Source: CAD feature listing. Evaluate the final solid. Frame: model axes, mm. Face numbers are marked on the shaded views. Coordinates: 2 decimals unless noted, no trailing zeros. Order: outer loops, then holes, each group sorted by start corner. A loop starts at its lowest first (then second) coordinate and runs counter-clockwise, first axis right, second up. Notation, with made-up numbers: (-12, 83) -> (1, 83) arc R11 ccw to (1, 87) -> close; hole circle Ø1 at (-15, -26). An arc over 180 degrees is marked (long way). Write item = value, one per line. Start each with the question number.
Item 1: Section query A-A (x = 0). Output: boundary loops of the cut face in (y, z).
Item 2: Contact query for flat-ended pins moving along their axis: pin 1 (5 mm diameter, centred on x = -3, y = 6.5, fed in from +Z); pin 2 (1.5 mm diameter, centred on x = 11, z = -13.5, fed in from -Y); pin 3 (3 mm diameter, centred on y = -3, z = -15.5, fed in from -X); pin 4 (6 mm diameter, centred on x = -13.5, z = -35, fed in from -Y). Output: stop coordinate, or through.
Item 3: Section query D-D (y = 0). Output: boundary loops of the cut face in (x, z).
Item 4: Mould query, pull axis X, two halves, no side actions, for the marked faces 1, 2 and 3. Classes: released by +X, released by -X, zero draft, split by the parting line, or undercut.
Item 5: Section query B-B (x = 24). Output: boundary loops of the cut face in (y, z), then the cut area to 3 significant figures.
Item 6: Ray query, line 1 along Y through (x, z) = (0, -54); line 2 along X through (y, z) = (12, -39); line 3 along X through (y, z) = (-4.5, -46). Return the intervals inside material, ascending. Write a range as [from, to].
Item 7: Section query C-C (z = -10). Output: boundary loops of the cut face in (x, y).
```python
from build123d import *

# Parameters (mm, degrees)
SKETCH4_W          = 60
SKETCH4_H          = 30
CUT_EXTRUDE1_REACH = 75.485
SKETCH6_W          = 42
SKETCH6_H          = 5
CIRPATTERN3_COUNT  = 6


with BuildPart() as part:
    # Sketch4 → Revolve1 (revolve)
    with BuildSketch(Plane(origin=(0, 0, 0), x_dir=(0, 0, -1), z_dir=(1, 0, 0)), mode=Mode.PRIVATE) as revolve1_sk:
        with Locations((30, 15)):
            Rectangle(SKETCH4_W, SKETCH4_H)
    revolve(revolve1_sk.sketch.rotate(Axis((0, 0, 24.398391619), (0, 0, -1)), 90), axis=Axis((0, 0, 24.398391619), (0, 0, -1)))

    # Sketch5 → Cut-Revolve1 (revolve, cut)
    with BuildSketch(Plane(origin=(0, 0, 0), x_dir=(0, 0, -1), z_dir=(1, 0, 0)), mode=Mode.PRIVATE) as cut_revolve1_sk:
        Polygon((0, 0), (0, 19.816349035), (50, 11), (60, 11), (60, 0), align=None)
    revolve(cut_revolve1_sk.sketch.rotate(Axis((0, 0, 8.48865663), (0, 0, -1)), 90), axis=Axis((0, 0, 8.48865663), (0, 0, -1)), mode=Mode.SUBTRACT)

    # Sketch6 → Cut-Extrude1 (cut, up to next)
    with BuildSketch(Plane(origin=(0, 0, 0), x_dir=(0, 0, -1), z_dir=(1, 0, 0)), mode=Mode.PRIVATE) as cut_extrude1_sk1:
        with Locations((21, 0)):
            Rectangle(SKETCH6_W, SKETCH6_H)
    cut_extrude1_tool1 = extrude(cut_extrude1_sk1.sketch, amount=CUT_EXTRUDE1_REACH, mode=Mode.PRIVATE) & part.part
    cut_extrude1 = cut_extrude1_tool1.solids().sort_by_distance((0, 0, -21))[0]
    add(cut_extrude1, mode=Mode.SUBTRACT)

    # CirPattern3: Cut-Extrude1 ×6 about axis
    cirpattern3_axis = Axis((0, 0, 0), (0, 0, 1))
    for i in range(1, CIRPATTERN3_COUNT):
        add(cut_extrude1.rotate(cirpattern3_axis, i * 360 / CIRPATTERN3_COUNT), mode=Mode.SUBTRACT)


solid = part.part
```
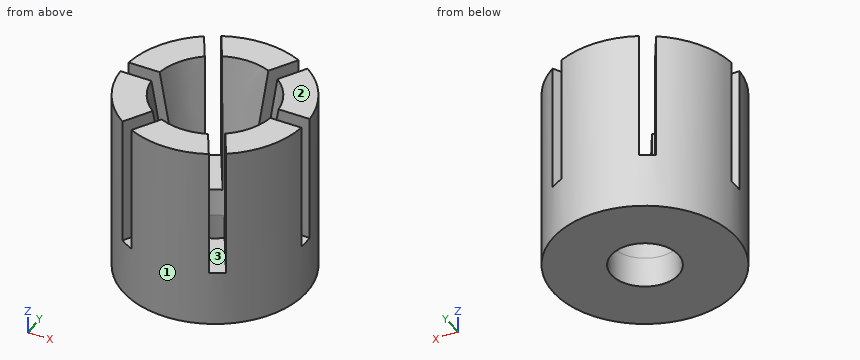
Computed:
q1.outline = (-30, -60) -> (-11, -60) -> (-11, -50) -> (-19.82, 0) -> (-30, 0) -> close; (11, -60) -> (30, -60) -> (30, 0) -> (19.82, 0) -> (11, -50) -> close
q2.pin_1 = through
q2.pin_2 = -28.19
q2.pin_3 = -29.9
q2.pin_4 = -28.1
q3.outline = (-30, -60) -> (-11, -60) -> (-11, -50) -> (-12.41, -42) -> (-30, -42) -> close; (11, -60) -> (30, -60) -> (30, -42) -> (12.41, -42) -> (11, -50) -> close
q4.face_1 = split by the parting line
q4.face_2 = zero draft
q4.face_3 = undercut
q5.outline = (-18, -60) -> (18, -60) -> (18, 0) -> (2.5, 0) -> (2.5, -42) -> (-2.5, -42) -> (-2.5, 0) -> (-18, 0) -> close
q5.area = 1,950 mm^2
q6.line_1 = [-30, -11], [11, 30]
q6.line_2 = [-27.5, -9.81], [9.81, 27.5]
q6.line_3 = [-29.66, -10.81], [10.81, 29.66]
q7.outline = (-29.9, -2.5) arc R30 ccw to (-17.11, -24.64) -> (-11.1, -14.23) arc R18.05 cw to (-17.88, -2.5) -> close; (-29.9, 2.5) -> (-17.88, 2.5) arc R18.05 cw to (-11.1, 14.23) -> (-17.11, 24.64) arc R30 ccw to start; (-12.78, -27.14) arc R30 ccw to (12.78, -27.14) -> (6.77, -16.73) arc R18.05 cw to (-6.77, -16.73) -> close; (-12.78, 27.14) -> (-6.77, 16.73) arc R18.05 cw to (6.77, 16.73) -> (12.78, 27.14) arc R30 ccw to start; (11.1, -14.23) -> (17.11, -24.64) arc R30 ccw to (29.9, -2.5) -> (17.88, -2.5) arc R18.05 cw to start; (11.1, 14.23) arc R18.05 cw to (17.88, 2.5) -> (29.9, 2.5) arc R30 ccw to (17.11, 24.64) -> close
